Input: part model. Units: mm. Frame: model coordinates. Coordinates: 2 decimals unless noted, no trailing zeros. Order: outer loops, then holes, each group sorted by start corner. A loop starts at its lowest first (then second) coordinate and runs counter-clockwise, first axis right, second up. Notation, with made-up numbers: M -38,2.25 L -32,2.25 A20 cw -32,7.25 Z; hole C 74.25,80.5 d8. An arc over 180 degrees is marked long. Answer in a Markdown table with one row per item.
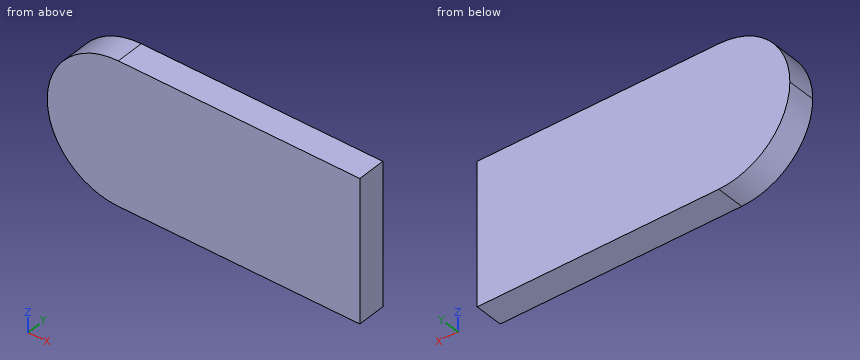
from build123d import *

# Parameters (mm, degrees)
F1_DEPTH = 5


with BuildPart() as f1:
    # F0 (on Front) → F1 (new body)
    with BuildSketch(Plane.XZ):
        with BuildLine():
            Line((0, 0), (-42.5, 0))
            ThreePointArc((-42.5, 0), (-51.338835, -3.661165), (-55, -12.5))
            ThreePointArc((-55, -12.5), (-51.338835, -21.338835), (-42.5, -25))
            Line((-42.5, -25), (0, -25))
            Line((0, -25), (0, 0))
        make_face()
    extrude(amount=F1_DEPTH)


solid = f1.part
1) Cut plane B-B, the plane x = -45. Output: boundary loops of the cut face in (y, z), and give its area (3 significant figures).
Resolved:
| item | result |
|---|---|
| outline | M -5,-24.75 L 0,-24.75 L 0,-0.25 L -5,-0.25 Z |
| area | 122 mm2 |
2) Material intervals for probe 1 along X at (y, z) = (-2.15, -23.5); probe 2 along Z at (x, y) = (-43, -0.7); probe 3 along X at (y, z) = (-2.55, -3.5), sorted ascending.
Resolved:
| item | result |
|---|---|
| probe 1 | x = -48.44 to 0 |
| probe 2 | z = -24.99 to -0.01 |
| probe 3 | x = -51.17 to 0 |
3) Cut plane C-C, the plane z = -21.25. Output: boundary loops of the cut face in (x, y).
Resolved:
| item | result |
|---|---|
| outline | M -51.43,-5 L 0,-5 L 0,0 L -51.43,0 Z |
4) Contact query for flat-ended pins moving along their axis: pin 1 (3 mm diameter, centred on y = -3, z = -20, fed in from -X); pin 2 (1 mm diameter, centred on x = -48, y = -3.5, fed in from -Z); pin 3 (1 mm diameter, centred on y = -3.5, z = -6.5, fed in from -X) (3 decimals). Output: stop coordinate, or through.
Resolved:
| item | result |
|---|---|
| pin 1 | stops at x = -53.47 |
| pin 2 | stops at z = -23.96 |
| pin 3 | stops at x = -53.725 |
5) Cut plane A-A, the plane y = -4. Output: boundary loops of the cut face in (x, z), and give its area (3 significant figures).
Resolved:
| item | result |
|---|---|
| outline | M -55,-12.5 A12.5 ccw -42.5,-25 L 0,-25 L 0,0 L -42.5,0 A12.5 ccw Z |
| area | 1,310 mm2 |
